```python
from build123d import *

# Parameters (mm, degrees)
Y_KSEKLIK_EKSTR_ZYON1_DEPTH      = 5
Y_KSEKLIK_EKSTR_ZYON1_DEPTH_BACK = 5
KES_EKSTR_ZYON1_DEPTH            = 10
IZIM3_R                          = 1.75
KES_EKSTR_ZYON2_DEPTH            = 7


with BuildPart() as part:
    # izim1 → Y_kseklik-Ekstr_zyon1 (new body, two sides)
    with BuildSketch(Plane(origin=(0, 0, 0), x_dir=(0, 0, -1), z_dir=(1, 0, 0))) as y_kseklik_ekstr_zyon1_sk:
        Polygon((-1.856187291, 5), (3.143812709, 5), (4, 1), (4, -5.5), (-4, -5.5), (-4, 1), align=None)
    extrude(amount=Y_KSEKLIK_EKSTR_ZYON1_DEPTH)
    extrude(y_kseklik_ekstr_zyon1_sk.sketch, amount=-Y_KSEKLIK_EKSTR_ZYON1_DEPTH_BACK)

    # izim2 → Kes-Ekstr_zyon1 (cut)
    with BuildSketch(Plane(origin=(0, 0, -4), x_dir=(-1, 0, 0), z_dir=(0, 0, -1))):
        Polygon((-3, -4.5), (-3, -5.5), (-2, -5.5), (-2, -4.5), (-0.5, -4.5), (-0.5, 0.5), (-4.5, 0.5), (-4.5, -4.5), align=None)
        Polygon((2, -4.5), (2, -5.5), (3, -5.5), (3, -4.5), (4.5, -4.5), (4.5, 0.5), (0.5, 0.5), (0.5, -4.5), align=None)
    extrude(amount=-KES_EKSTR_ZYON1_DEPTH, mode=Mode.SUBTRACT)

    # izim3 → Kes-Ekstr_zyon2 (cut)
    with BuildSketch(Plane(origin=(0, 5, 0), x_dir=(1, 0, 0), z_dir=(0, 1, 0))):
        with Locations((-2.5, 0.643812709)):
            Circle(IZIM3_R)
        with Locations((2.5, 0.643812709)):
            Circle(IZIM3_R)
    extrude(amount=-KES_EKSTR_ZYON2_DEPTH, mode=Mode.SUBTRACT)


solid = part.part
```
Geometry check sheet. Reference: the model listing, model coordinates, mm. A direction names the side the tool comes from. Coordinates: 2 decimals unless noted, no trailing zeros. Order: outer loops, then holes, each group sorted by start corner. A loop starts at its lowest first (then second) coordinate and runs counter-clockwise, first axis right, second up.
Item 1: Section check C-C (z = -2.25). Enter the section's corners in (x, y), plus the area to 3 significant figures.
Item 2: Depth check by flat-ended pin: pin 1 (4.5 mm diameter, centred on x = -2.5, z = -0.64, fed in from +Y). Enter the tip coordinate at first touch or a pass-through.
Item 3: Section check B-B (x = -3.25). Enter the section's corners in (y, z), plus the area to 3 significant figures.
Item 4: Section check A-A (y = 0). Enter the section's corners in (x, z).
Item 5: Scan lines: line 1 along X through (y, z) = (-2.75, 1.25); line 2 along Y through (x, z) = (-1, 1.25); line 3 along X through (y, z) = (2, -0.75). Record each from-to range of solid material in increasing order.
Item 6: Tool access check on faces 3 (the flat face through (0, -5.5, 0)), 4 (the flat face through (4, 0.5, 1)), 5 (the cylindrical face through (4.117, 2.782, 0.026)), 6 (the flat face through (0, -2, 4)), 7 (the flat face through (-3, -5, 0)). Record the directions out of +Z, -Z, +X, -X, +Y, -Y that give a thin tool (end or side, any length) a straight path to the whole face; none if there is none.
Item 7: Mould release check, pull along X, two halves, no side actions. Record for faces 1 (the flat face through (4.5, -2, 0)), 2 (the flat face through (0.07, 2.972, 2.943)): released by +X, released by -X, zero draft, split by the parting line, or undercut.
Item 8: Section check D-D (x = 2.5). Enter the section's corners in (y, z).
Check sheet entries:
1. outline: (-5, -5.5) - (-3, -5.5) - (-3, -4.5) - (-4.5, -4.5) - (-4.5, 0.5) - (-3.19, 0.5) - (-3.19, 5) - (-5, 5) - close; (-2, -5.5) - (2, -5.5) - (2, -4.5) - (0.5, -4.5) - (0.5, 0.5) - (1.81, 0.5) - (1.81, 5) - (-1.81, 5) - (-1.81, 0.5) - (-0.5, 0.5) - (-0.5, -4.5) - (-2, -4.5) - close; (3, -5.5) - (5, -5.5) - (5, 5) - (3.19, 5) - (3.19, 0.5) - (4.5, 0.5) - (4.5, -4.5) - (3, -4.5) - close
1. area: 50.5 mm2
2. pin 1: stops at y = 5
3. outline: (-5.5, -4) - (-4.5, -4) - (-4.5, 4) - (-5.5, 4) - close; (0.5, -4) - (1, -4) - (5, -3.14) - (5, -2.22) - (0.5, -2.22) - close; (0.5, 0.94) - (5, 0.94) - (5, 1.86) - (1, 4) - (0.5, 4) - close
3. area: 23.8 mm2
4. outline: (-5, -4) - (-4.5, -4) - (-4.5, 4) - (-5, 4) - close; (-0.5, -4) - (0.5, -4) - (0.5, 4) - (-0.5, 4) - close; (4.5, -4) - (5, -4) - (5, 4) - (4.5, 4) - close
5. line 1: x = -5 to -4.5, -0.5 to 0.5, 4.5 to 5
5. line 2: y = -5.5 to -4.5, 0.5 to 5
5. line 3: x = -5 to -4.25, -0.75 to 0.75, 4.25 to 5
6. face 3: +Z, -Z, +X, -X, -Y
6. face 4: +Z, -Z
6. face 5: +Y
6. face 6: +Z, +X, -X, +Y, -Y
6. face 7: +Z, -Z, -Y
7. face 1: undercut
7. face 2: zero draft
8. outline: (0.5, -4) - (1, -4) - (5, -3.14) - (5, -2.39) - (0.5, -2.39) - close; (0.5, 1.11) - (5, 1.11) - (5, 1.86) - (1, 4) - (0.5, 4) - close
